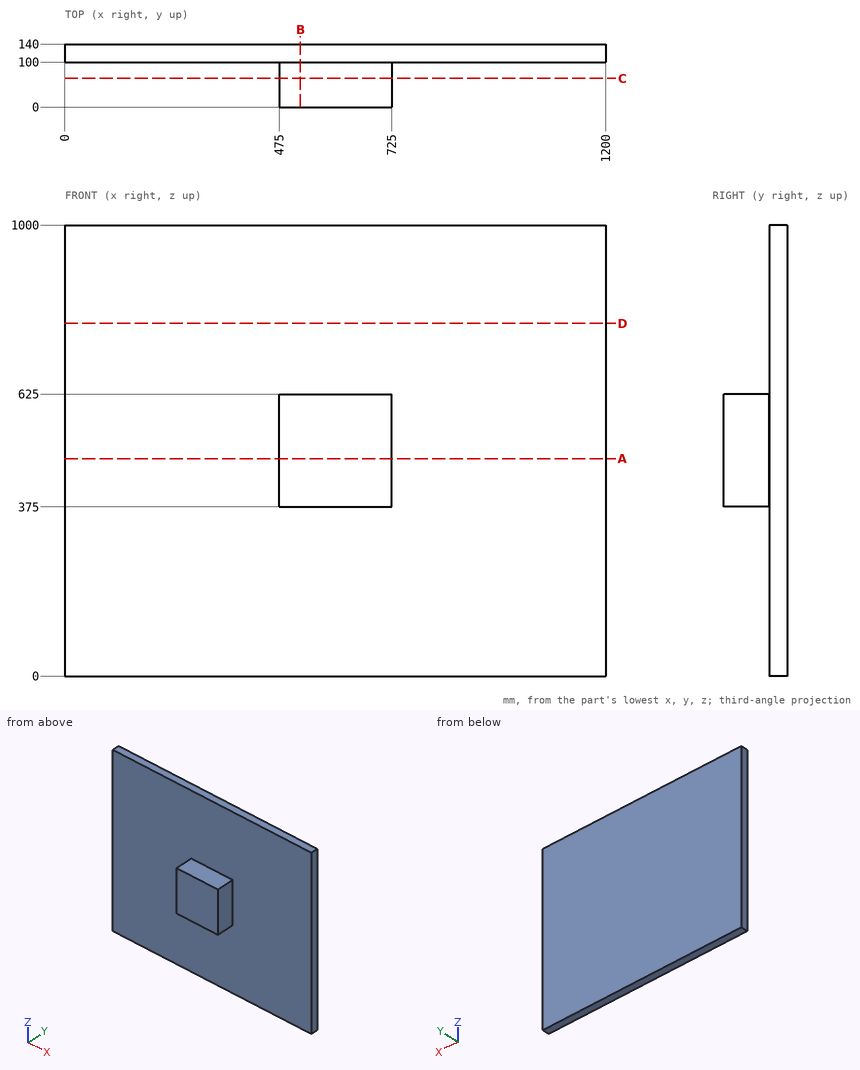
Drawing for the job (mm, zero at the part's lowest x, y, z). Coordinates: 2 decimals unless noted, no trailing zeros. Write each loop counter-clockwise with the first axis right and the second up, starting at its lowest first coordinate (ties: lowest second). Pieces come first, ordered by that corner, then holes. Notation, with made-up numbers: (87, 61.25) - (108, 61.25) arc R30 cw to (108, 99.25) - close; hole circle Ø7 at (18, 40). An arc over 180 degrees is marked (long way). Write each question's results on one line, items separated by ' | '. Start each with the question number.
1) Cut at B-B (x = 522). Write the cut outline in (y, z).
2) Cut at D-D (z = 782). Write the cut outline in (x, y), then the cut area to 3 significant figures.
3) Flat gauge pins, fed straight in: P1, Ø6, axis at y = 43, z = 408.5, coming from the -X side; P2, Ø2, axis at y = 97, z = 524.5, coming from the +X side; P3, Ø2, axis at x = 221.5, z = 685.5, coming from the -Y side. Where does each tip first touch, or does it go through?
4) Probe line 1 along Y through (x, z) = (114, 858); line 2 along Z through (x, y) = (499, 13.5); line 3 along X through (y, z) = (92.5, 578). List the from-to ranges inside material, lowest first. Write a range as from..to.
5) Cut at A-A (z = 482). Write the cut outline in (x, y), then the cut area to 3 significant figures.
6) Cut at C-C (y = 63.5). Write the cut outline in (x, z).
Returned:
1) outline: (0, 375) - (100, 375) - (100, 0) - (140, 0) - (140, 1000) - (100, 1000) - (100, 625) - (0, 625) - close
2) outline: (0, 100) - (1200, 100) - (1200, 140) - (0, 140) - close | area: 48,000 mm^2
3) P1: x = 475 | P2: x = 725 | P3: y = 100
4) line 1: 100..140 | line 2: 375..625 | line 3: 475..725
5) outline: (0, 100) - (475, 100) - (475, 0) - (725, 0) - (725, 100) - (1200, 100) - (1200, 140) - (0, 140) - close | area: 73,000 mm^2
6) outline: (475, 375) - (725, 375) - (725, 625) - (475, 625) - close
